Geometry check sheet. Reference: the model listing, model coordinates, mm. A direction names the side the tool comes from. Give positions to 0.01 mm unless a question says otherwise; leave off trailing zeros. Loops run counter-clockwise (first coordinate to the right, second up) from the corner with the lowest first, then second, coordinate; pieces in that order, holes last. Notation, with made-up numbers: (46.5, 86.25) -> (85.5, 86.25) arc R20 cw to (85.5, 100.25) -> close; hole circle Ø4 at (64, 3). An arc over 180 degrees is marked (long way). Answer in a Markdown table with one row per item. Add a question column.
Autodesk Inventor part; units mm, degrees
ref_plane "YZ Plane" through (0, 0, 0) normal (1, 0, 0) x (0, 1, 0)
ref_plane "XZ Plane" through (0, 0, 0) normal (0, 1, 0) x (-1, 0, 0)
ref_plane "XY Plane" through (0, 0, 0) normal (0, 0, 1) x (1, 0, 0)
sketch "Sketch1" plane through (0, 0, 0) normal (0, 1, 0) x (-1, 0, 0)
  line L0 (0, 0) -> (0, -250)
  line L1 (-200, 0) -> (0, 0)
  line L2 (0, -250) -> (0, -300)
  line L3 (0, -300) -> (-200, -300)
  line L4 (-200, -300) -> (-230, -300)
  line L5 (-230, 0) -> (-200, 0)
  line L6 (-230, -300) -> (-245, -300)
  line L7 (-245, -300) -> (-245, 0)
  line L8 (-245, 0) -> (-230, 0)
  dimension "d0" = 250
  dimension "d4" = 50
  dimension "d12" = 30
  dimension "d24" = 15
extrude "Extrusion1" add sketch "Sketch1" along normal blind 38
sketch "Sketch2" plane through (0, 38, 0) normal (0, 1, 0) x (1, 0, 0)
  line L0 (0, 300) -> (0, 0)
  line L1 (0, 0) -> (245, 0)
  line L2 (10, 10) -> (10, 290)
  line L3 (245, 300) -> (0, 300)
  line L4 (245, 0) -> (245, 300)
  line L5 (245, 290) -> (235, 290)
  line L6 (235, 290) -> (235, 10)
  line L7 (235, 290) -> (10, 290)
  line L8 (0, 300) -> (0, 0)
  line L9 (235, 10) -> (10, 10)
  dimension "d25" = 10
extrude "Extrusion2" cut sketch "Sketch2" against normal blind 30 contours L2 L7 L6 L9
move faces "Move1" translate (0, 0, -84.138) faces at (81.6667, 25.3333, 0)
move faces "Move2" translate (-15.875, 0, 0) faces at (245, 25.3333, -156.092)
sketch "Sketch15" plane through (0, 8, 0) normal (0, 1, 0) x (1, 0, 0)
  line L0 (10, 84.138) -> (10, 290)
  line L1 (10, 84.138) -> (10, 94.138)
  line L2 (10, 94.138) -> (219.125, 94.138)
  line L3 (229.125, 290) -> (229.125, 84.138)
  line L4 (229.125, 290) -> (219.125, 290)
  line L5 (10, 290) -> (229.125, 290)
  line L6 (219.125, 290) -> (219.125, 94.138)
  line L7 (10, 84.138) -> (229.125, 84.138)
  line L8 (229.125, 290) -> (229.125, 84.138)
  point P0 (0, 0)
  dimension "d42" = 10
  dimension "d43" = 10
extrude "Extrusion5" add sketch "Sketch15" along normal blind 30 contours L0 L2 L6 L4 L3 L7
sketch "Sketch16" plane through (229.125, 0, -84.138) normal (1, 0, 0) x (0, 0, -1)
  line L0 (10, 8) -> (205.862, 8)
  line L1 (155.5172, 8) -> (155.5172, 38)
  line L2 (215.862, 38) -> (0, 38)
  circle A0 centre (155.5172, 23) radius 13.5
  point P0 (-84.138, 0)
  dimension "d46" = 27
extrude "Extrusion6" cut sketch "Sketch16" against normal blind 235
equation "\"BendRadius\" = Thickness"
equation "\"BendReliefWidth\" = Thickness"
equation "\"BendReliefDepth\" = 0.5 * Thickness"
equation "\"CornerReliefSize\" = 4 * Thickness"
equation "\"MinimumRemnant\" = 2 * Thickness"
equation "\"TransitionRadius\" = BendRadius"
equation "\"JacobiRadiusSize\" = BendRadius"
equation "\"GapSize\" = Thickness"
properties part number "Case_3d_model_3DPrint"
1. Access from +Z, -Z, +X, -X, +Y, -Y to the whole of each face (thin tool, end or side, straight path). Record for faces 1 (the face through (113, 8, -193)), 2 (the face through (0, 19, -191)).
2. Sectioned sample at D-D (z = -242). Enter the section's corners in (x, y) (3 decimals).
3. Sectioned sample at B-B (x = 118). Enter the section's corners in (y, z), plus the area to 3 significant figures.
4. Gauge pin test, flat end, axial feed: pin 1 Ø8 at (x, z) = (84.5, -210.5) entering from +Y. Record the tip position at first contact, or that the pin passes through.
5. Material ranges on L1, parallel to Z at x = 210, y = 20.5; L2, parallel to Z at x = 222, y = 23; L3, parallel to X at y = 20, z = -199 (3 decimals), recorded low to high. Write a range as from..to.
6. Sectioned sample at C-C (z = -173). Enter the section's corners in (x, y) (3 decimals).
7. Sectioned sample at A-A (y = 23). Enter the section's corners in (x, z) (3 decimals).
8. Release check for a two-part mould opening along Y. For faces 3 (the face through (124, 38, -295)), 4 (the face through (224.195, 17.829, -252.126)), 5 (the face through (5.07, 17.829, -252.126)), 6 (the face through (113, 19, -300)) record: released by +Y, released by -Y, zero draft, split by the parting line, or undercut.
Response:
| question | item | result |
|---|---|---|
| 1 | face 1 | +Y |
| 1 | face 2 | +Z, -Z, -X, +Y, -Y |
| 2 | outline | (0, 0) -> (229.125, 0) -> (229.125, 9.705) -> (219.125, 9.705) -> (219.125, 8) -> (10, 8) -> (10, 9.705) -> (0, 9.705) -> close; (0, 36.295) -> (10, 36.295) -> (10, 38) -> (0, 38) -> close; (219.125, 36.295) -> (229.125, 36.295) -> (229.125, 38) -> (219.125, 38) -> close |
| 3 | outline | (0, -300) -> (38, -300) -> (38, -290) -> (8, -290) -> (8, -94.14) -> (38, -94.14) -> (38, -84.14) -> (0, -84.14) -> close |
| 3 | area | 2,330 mm2 |
| 4 | pin 1 | stops at y = 8 |
| 5 | L1 | z = -300..-290, -94.14..-84.14 |
| 5 | L2 | z = -300..-253.16, -226.16..-84.14 |
| 5 | L3 | x = 0..10, 219.125..229.125 |
| 6 | outline | (0, 0) -> (229.125, 0) -> (229.125, 38) -> (219.125, 38) -> (219.125, 8) -> (10, 8) -> (10, 38) -> (0, 38) -> close |
| 7 | outline | (0, -300) -> (229.125, -300) -> (229.125, -253.155) -> (219.125, -253.155) -> (219.125, -290) -> (10, -290) -> (10, -253.155) -> (0, -253.155) -> close; (0, -226.155) -> (10, -226.155) -> (10, -94.138) -> (219.125, -94.138) -> (219.125, -226.155) -> (229.125, -226.155) -> (229.125, -84.138) -> (0, -84.138) -> close |
| 8 | face 3 | released by +Y |
| 8 | face 4 | undercut |
| 8 | face 5 | undercut |
| 8 | face 6 | zero draft |
